Verification items for the finished model (mm, model axes). A direction names the side the tool comes from. Give positions to 0.01 mm unless a question says otherwise; leave off trailing zeros. Loops run counter-clockwise (first coordinate to the right, second up) from the corner with the lowest first, then second, coordinate; pieces in that order, holes last. Notation, with made-up numbers: (61, 45) - (117, 45) arc R20 ccw to (117, 83) - close; hole circle Ø7 at (-27.5, 63). An arc over 180 degrees is marked (long way). Answer in a Markdown table with one row per item.
```python
from build123d import *

# Parameters (mm, degrees)
F0_R     = 31.5738283612
F1_DEPTH = 78.994
F3_D     = 6.6
F5_W     = 42.1696881435
F5_H     = 47.0036589152
F5_R     = 3.3
F6_DEPTH = 37.846
F7_SIZE2 = 5.08
F7_SIZE  = 5.08
F8_F1_R  = 5.08
F8_F2_R  = 5.08
F8_F3_R  = 5.0799
F8_F4_R  = 5.0799
F9_SIZE  = 2.54
F10_SIZE = 5.08


# Not quite as in the source:
# - a fillet or chamfer is up to 0.001 mm smaller than in the source, because OpenCascade refuses the exact size


with BuildPart() as f1:
    # F0 (on Front) → F1 (new body)
    with BuildSketch(Plane.XZ):
        Circle(F0_R)
    extrude(amount=F1_DEPTH)

    # F3 (through all)
    with Locations(Plane.XZ.offset(78.994)):
        with Locations((0, 0)):
            Hole(F3_D / 2)

    # F5 (on face) → F6 (join)
    with BuildSketch(Plane(origin=(0, 0, 0), x_dir=(-1, 0, 0), z_dir=(0, 1, 0))):
        Rectangle(F5_W, F5_H)
        Circle(F5_R, mode=Mode.SUBTRACT)
    extrude(amount=F6_DEPTH)

    # F7
    f7_edges = [f1.edges().sort_by_distance(p)[0] for p in [
        (21.084844, 18.923, 23.501829),
        (21.084844, 18.923, -23.501829),
        (-21.084844, 18.923, 23.501829),
        (-21.084844, 18.923, -23.501829),
    ]]
    chamfer(f7_edges, length=F7_SIZE, length2=F7_SIZE2)

    # F8: fillet of radius 5.08 on 4 edges, made by hand

    # F8_f1
    f8_f1_edges = [f1.edges().sort_by_distance(p)[0] for p in [
        (-21.0848440718, 37.846, 0),
    ]]
    fillet(f8_f1_edges, radius=F8_F1_R)

    # F8_f2
    f8_f2_edges = [f1.edges().sort_by_distance(p)[0] for p in [
        (21.0848440718, 37.846, 0),
    ]]
    fillet(f8_f2_edges, radius=F8_F2_R)

    # F8_f3 (radius 5.08 in the source; OpenCascade refuses exactly that, so slightly less here)
    f8_f3_edges = [f1.edges().sort_by_distance(p)[0] for p in [
        (0, 37.846, -23.5018294576),
    ]]
    fillet(f8_f3_edges, radius=F8_F3_R)

    # F8_f4 (radius 5.08 in the source; OpenCascade refuses exactly that, so slightly less here)
    f8_f4_edges = [f1.edges().sort_by_distance(p)[0] for p in [
        (0, 37.846, 23.5018294576),
    ]]
    fillet(f8_f4_edges, radius=F8_F4_R)

    # F9
    f9_edges = [f1.edges().sort_by_distance(p)[0] for p in [
        (-31.573828, 0, 0),
    ]]
    chamfer(f9_edges, length=F9_SIZE)

    # F10
    f10_edges = [f1.edges().sort_by_distance(p)[0] for p in [
        (-31.573828, -78.994, 0),
    ]]
    chamfer(f10_edges, length=F10_SIZE)


solid = f1.part
```
Q1. Go/stop test with flat-tipped pins: P1, Ø16.5, axis at y = 11.5, z = 0.5, coming from the -X side; P2, Ø3, axis at x = -22, y = 12, coming from the -Z side; P3, Ø1, axis at y = -1.5, z = 18, coming from the -X side. Record where each tip stops, or that it passes through.
Completed:
| item | result |
|---|---|
| P1 | x = -21.08 |
| P2 | z = -19.01 |
| P3 | x = -25.37 |
Q2. Tool access check on faces 1 (the face through (-21.085, 16, 0)), 2 (the face through (-18.58, 18.323, 20.926)), 3 (the face through (18.509, 18.323, -20.997)), 4 (the face through (21.085, 16, 0)), 5 (the face through (0, 16, -23.502)). Record the directions out of +Z, -Z, +X, -X, +Y, -Y that give a thin tool (end or side, any length) a straight path to the whole face; none if there is none.
Completed:
| item | result |
|---|---|
| face 1 | +Z, -Z, -X, +Y |
| face 2 | +Z, -X, +Y |
| face 3 | -Z, +X, +Y |
| face 4 | +Z, -Z, +X, +Y |
| face 5 | -Z, +X, -X, +Y |
Q3. Thickness scan on line 1 (Z direction, x = 0, y = -43); line 2 (Z direction, x = 0, y = 21); line 3 (X direction, y = 21, z = 16). Record the ranges inside material, lowest first.
Completed:
| item | result |
|---|---|
| line 1 | -31.57 to -3.3, 3.3 to 31.57 |
| line 2 | -23.5 to -3.3, 3.3 to 23.5 |
| line 3 | -21.08 to 21.08 |
Q4. Sectioned sample at A-A (y = 28.5). Record the cut outline in (x, z), and give its area (3 significant figures).
Completed:
| item | result |
|---|---|
| outline | (-21.08, -18.42) - (-16, -23.5) - (16, -23.5) - (21.08, -18.42) - (21.08, 18.42) - (16, 23.5) - (-16, 23.5) - (-21.08, 18.42) - close; hole circle Ø6.6 at (0, 0) |
| area | 1,900 mm^2 |
Q5. Sectioned sample at B-B (y = -50.5). Record the cut outline in (x, z).
Completed:
| item | result |
|---|---|
| outline | circle Ø63.15 at (0, 0); hole circle Ø6.6 at (0, 0) |
